Design review of the part built by this model. Coordinates are the model's own, in mm. Give positions to 0.01 mm unless a question says otherwise; leave off trailing zeros. Loops run counter-clockwise (first coordinate to the right, second up) from the corner with the lowest first, then second, coordinate; pieces in that order, holes last. Notation, with made-up numbers: (75.25, 15.25) -> (127.25, 15.25) arc R9 ccw to (127.25, 31.25) -> close; hole circle Ø4 at (19, 19.5). An arc over 180 degrees is marked (long way). Use CSV: the item, a comma, the result in double quotes. Start each with the question number.
Item 1: We need section A-A (z = 1.9). State the section outline as (x, y) points.
Item 2: Wall thickness on line 1 along Y through (x, z) = (-88.5, 2.35); line 2 along Y through (x, z) = (38, 0.2); line 3 along X through (y, z) = (33.5, 0.95): over which ranges is each line inside the solid? List them lowest first. Write a range as from..to.
Item 3: We need section C-C (x = -78). State the section outline as (y, z) points, plus the area to 3 significant figures.
Item 4: We need section B-B (y = 31). State the section outline as (x, z) points, plus the area to 3 significant figures.
Item 5: Clearance check with a flat-ended pin moving along its axis: pin 1 (0.8 mm diameter, centred on x = 89, y = -55, fed in from +Z). State where the tip first meets the part, or that it passes through.
from build123d import *

# Parameters (mm, degrees)
SKETCH_1_W          = 181.2
SKETCH_1_H          = 116
EXTRUDE_1_DEPTH     = 1
SKETCH_2_R          = 2
SKETCH_2_R_2        = 1.25
EXTRUDE_2_DEPTH     = 3
SKETCH_3_W          = 163
SKETCH_3_H          = 97
CUT_EXTRUDE_2_DEPTH = 3


with BuildPart() as part:
    # 草图1 → 凸台-拉伸1 (new body)
    with BuildSketch(Plane.XY):
        Rectangle(SKETCH_1_W, SKETCH_1_H)
    extrude(amount=EXTRUDE_1_DEPTH)

    # 草图2 → 凸台-拉伸2 (add)
    # profile 1 of 4: a face of its own
    with BuildSketch(Plane.XY.offset(1)):
        with Locations((-88.5, 55)):
            Circle(SKETCH_2_R)
        with Locations((-88.5, 55)):
            Circle(SKETCH_2_R_2, mode=Mode.SUBTRACT)
    # profile 2 of 4: a face of its own
    with BuildSketch(Plane.XY.offset(1)):
        with Locations((88.5, 55)):
            Circle(SKETCH_2_R)
        with Locations((88.5, 55)):
            Circle(SKETCH_2_R_2, mode=Mode.SUBTRACT)
    # profile 3 of 4: a face of its own
    with BuildSketch(Plane.XY.offset(1)):
        with Locations((88.5, -55)):
            Circle(SKETCH_2_R)
        with Locations((88.5, -55)):
            Circle(SKETCH_2_R_2, mode=Mode.SUBTRACT)
    # profile 4 of 4: a face of its own
    with BuildSketch(Plane.XY.offset(1)):
        with Locations((-88.5, -55)):
            Circle(SKETCH_2_R)
        with Locations((-88.5, -55)):
            Circle(SKETCH_2_R_2, mode=Mode.SUBTRACT)
    extrude(amount=EXTRUDE_2_DEPTH)

    # 草图3 → 切除-拉伸2 (cut)
    with BuildSketch(Plane(origin=(0, 0, 0), x_dir=(-1, 0, 0), z_dir=(0, 0, -1))):
        Rectangle(SKETCH_3_W, SKETCH_3_H)
    extrude(amount=-CUT_EXTRUDE_2_DEPTH, mode=Mode.SUBTRACT)


solid = part.part
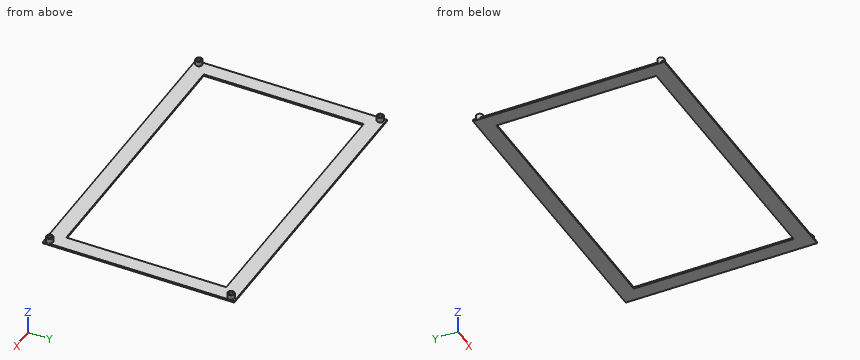
Results found:
1,outline,"circle Ø4 at (-88.5, -55); circle Ø4 at (-88.5, 55); circle Ø4 at (88.5, -55); circle Ø4 at (88.5, 55); hole circle Ø2.5 at (-88.5, -55); hole circle Ø2.5 at (-88.5, 55); hole circle Ø2.5 at (88.5, -55); hole circle Ø2.5 at (88.5, 55)"
2,line 1,"-57..-56.25, -53.75..-53, 53..53.75, 56.25..57"
2,line 2,"-58..-48.5, 48.5..58"
2,line 3,"-90.6..-81.5, 81.5..90.6"
3,outline,"(-58, 0) -> (-48.5, 0) -> (-48.5, 1) -> (-58, 1) -> close; (48.5, 0) -> (58, 0) -> (58, 1) -> (48.5, 1) -> close"
3,area,"19.0 mm²"
4,outline,"(-90.6, 0) -> (-81.5, 0) -> (-81.5, 1) -> (-90.6, 1) -> close; (81.5, 0) -> (90.6, 0) -> (90.6, 1) -> (81.5, 1) -> close"
4,area,"18.2 mm²"
5,pin 1,"z = 1"
